```python
from build123d import *

# Parameters (mm, degrees)
F0_W     = 65
F0_H     = 60
F1_DEPTH = 2.54
F2_R     = 1.27
F3_DEPTH = 2.541
F4_W     = 3.186375
F4_H     = 6.750785
F5_DEPTH = 3.5


with BuildPart() as f1:
    # F0 (on Top) → F1 (new body)
    with BuildSketch(Plane.XY):
        with Locations((53.585585, -131.870539)):
            Rectangle(F0_W, F0_H)
    extrude(amount=F1_DEPTH)

    # F2 (on face) → F3 (cut, through all)
    with BuildSketch(Plane.XY.offset(2.54)):
        with Locations((24.260585, -105.045539)):
            Circle(F2_R)
        with Locations((82.910585, -105.045539)):
            Circle(F2_R)
        with Locations((82.910585, -158.695539)):
            Circle(F2_R)
        with Locations((24.260585, -158.695539)):
            Circle(F2_R)
    extrude(amount=-F3_DEPTH, mode=Mode.SUBTRACT)

    # F4 (on face) → F5 (join)
    with BuildSketch(Plane.XY.offset(2.54)):
        with Locations((74.301257, -103.201653)):
            Rectangle(F4_W, F4_H)
    extrude(amount=F5_DEPTH)


solid = f1.part
```
Input: part model. Units: mm. Frame: model coordinates. A direction names the side the tool comes from. Coordinates: 2 decimals unless noted, no trailing zeros. Loops run counter-clockwise (first coordinate to the right, second up) from the corner with the lowest first, then second, coordinate; pieces in that order, holes last. Notation, with made-up numbers: (1.5, 46) - (40.5, 46) arc R8 cw to (40.5, 55) - close; hole circle Ø10 at (-24, 84.25). An arc over 180 degrees is marked (long way). Answer in a Markdown table with one row per item.
(1) Mould query, pull axis Y, two halves, no side actions, for faces 6 (the face through (82.745, -103.786, 1.288)), 7 (the face through (24.095, -103.786, 1.288)), 8 (the face through (74, -106.577, 4)), 9 (the face through (86.086, -132, 1)). Classes: pulls with the +Y half, pulls with the -Y half, needs draft (parallel to the pull), parting line crosses it, or undercut.
Model answer:
| item | result |
|---|---|
| face 6 | undercut |
| face 7 | undercut |
| face 8 | pulls with the -Y half |
| face 9 | needs draft |
(2) Cut plane C-C on x = 34. Output: boundary loops of the cut face in (y, z).
Model answer:
| item | result |
|---|---|
| outline | (-161.87, 0) - (-101.87, 0) - (-101.87, 2.54) - (-161.87, 2.54) - close |
(3) Material intervals for L1, parallel to X at y = -159, z = 1.75; L2, parallel to Y at x = 82.5, z = 2.25; L3, parallel to Z at x = 80, y = -131, sorted ascending. Write a range as from..to.
Model answer:
| item | result |
|---|---|
| L1 | x = 21.09..23.03, 25.49..81.68, 84.14..86.09 |
| L2 | y = -161.87..-159.9, -157.49..-106.25, -103.84..-101.87 |
| L3 | z = 0..2.54 |
(4) Cut plane A-A on z = 1.5. Output: boundary loops of the cut face in (x, y), plus the area to 3 significant figures.
Model answer:
| item | result |
|---|---|
| outline | (21.09, -161.87) - (86.09, -161.87) - (86.09, -101.87) - (21.09, -101.87) - close; hole circle Ø2.54 at (24.26, -158.7); hole circle Ø2.54 at (24.26, -105.05); hole circle Ø2.54 at (82.91, -158.7); hole circle Ø2.54 at (82.91, -105.05) |
| area | 3,880 mm² |
(5) Cut plane B-B on y = -139. Output: boundary loops of the cut face in (x, z).
Model answer:
| item | result |
|---|---|
| outline | (21.09, 0) - (86.09, 0) - (86.09, 2.54) - (21.09, 2.54) - close |
(6) Pin query (flat end, axial travel): P1, Ø2, axis at x = 78.5, z = 5, coming from the -Y side; P2, Ø1.5, axis at x = 41.5, y = -154.5, coming from the +Z side; P3, Ø1, axis at x = 74.5, z = 3.5, coming from the -Y side; P4, Ø1, axis at x = 74.5, y = -101, coming from the -Z side. Return the tip coordinate at first contact, or that it passes through.
Model answer:
| item | result |
|---|---|
| P1 | passes through |
| P2 | stops at z = 2.54 |
| P3 | stops at y = -106.58 |
| P4 | stops at z = 2.54 |
(7) Set-up query: faces 1 (the face through (75.894, -103, 4)), 2 (the face through (23.985, -159.935, 1.288)), 3 (the face through (74, -101, 2.54)), 4 (the face through (72.708, -103, 4)), 5 (the face through (74, -99.826, 4)). Return all of +Z, -Z, +X, -X, +Y, -Y with unobstructed straight access to the full face (end or side cutting, diameter ignored); none if empty.
Model answer:
| item | result |
|---|---|
| face 1 | +Z, +X, +Y, -Y |
| face 2 | +Z, -Z |
| face 3 | -Z, +X, -X, +Y |
| face 4 | +Z, -X, +Y, -Y |
| face 5 | +Z, -Z, +X, -X, +Y |
